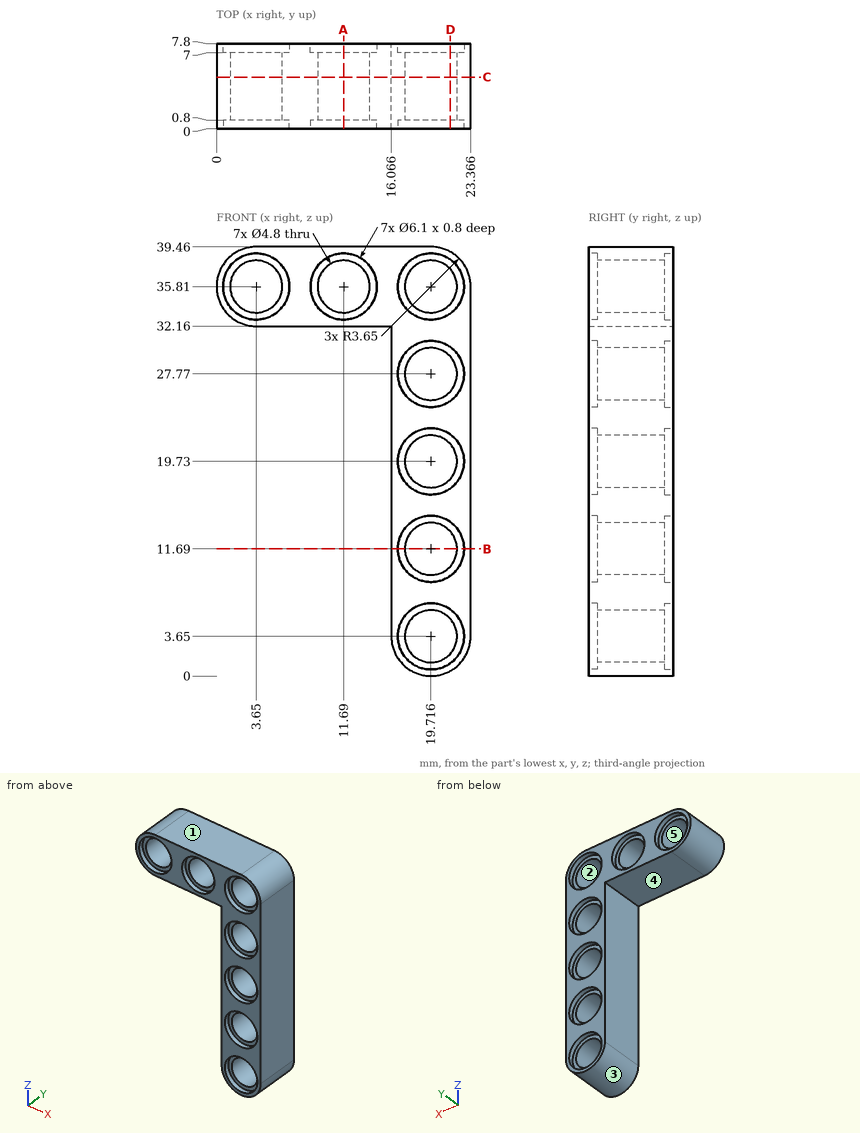
Answer from the drawing. Dimensions are ordinates in mm from the lowest x, y and z of the part. A direction names the side the tool comes from. Give positions to 0.01 mm unless a question says otherwise; leave off trailing zeros. Loops run counter-clockwise (first coordinate to the right, second up) from the corner with the lowest first, then second, coordinate; pieces in that order, holes last. Notation, with made-up numbers: (-16, 2.5) - (18, 2.5) arc R14 ccw to (18, 13.5) - close; hole circle Ø5 at (66.25, 85.5). An arc over 180 degrees is marked (long way). Answer as CSV lines item,"result". Start each with the question number.
Item 1: For the marked faces 4 and 5, determine the directions among +Z, -Z, +X, -X, +Y, -Y from which every point of the face is accessible in a straight line to the end or side of a thin tool.
Item 2: A cutting plane is placed at D-D on x = 21.5. Count the separate pieces of the cut face and the enclosed holes in it, then the cut area to 3 significant figures.
Item 3: A cutting plane is placed at B-B on z = 11.69. Determine the outline of the cut face in (x, y).
Item 4: The mould has two halves that part along X. Classify the marked faces 1, 2 and 3: +X half, -X half, draft (parallel to the pull), parting line (faces both ways), or undercut.
Item 5: A cutting plane is placed at C-C on y = 4.75. Determine the outline of the cut face in (x, z), then the cut area to 3 significant figures.
Item 6: A cutting plane is placed at A-A on x = 11.69. Determine the outline of the cut face in (y, z).
Item 7: Find the intervals of material crossed by line 1 (X direction, y = 7.5, z = 35.81); line 2 (Z direction, x = 11.69, y = 2); line 3 (X direction, y = 7.3, z = 11.69), in increasing order. Write a range as from..to.
Item 8: Each of these flat-tipped pins is pushed along its axis until it touches: pin 1 (1.8 mm diameter, centred on x = 18.5, z = 37, fed in from -Y); pin 2 (3.5 mm diameter, centred on x = 19.72, z = 19.73, fed in from +Y); pin 3 (5 mm diameter, centred on x = 3.65, z = 35.81, fed in from +Y); pin 4 (2 mm diameter, centred on x = 16.5, y = 1, fed in from -Z). Where does it stop, or does it pass through?
Found:
1,face 4,"-Z, -X, +Y, -Y"
1,face 5,"+Y, -Y"
2,separate pieces,"6"
2,enclosed holes,"0"
2,area,"161 mm^2"
3,outline,"(16.07, 0) - (16.67, 0) - (16.67, 0.8) - (17.32, 0.8) - (17.32, 7) - (16.67, 7) - (16.67, 7.8) - (16.07, 7.8) - close; (22.12, 0.8) - (22.77, 0.8) - (22.77, 0) - (23.37, 0) - (23.37, 7.8) - (22.77, 7.8) - (22.77, 7) - (22.12, 7) - close"
4,face 1,"draft"
4,face 2,"undercut"
4,face 3,"parting line"
5,outline,"(3.65, 32.16) - (16.07, 32.16) - (16.07, 3.65) arc R3.65 ccw to (23.37, 3.65) - (23.37, 35.81) arc R3.65 ccw to (19.72, 39.46) - (3.65, 39.46) arc R3.65 ccw to start; hole circle Ø4.8 at (3.65, 35.81); hole circle Ø4.8 at (11.69, 35.81); hole circle Ø4.8 at (19.72, 3.65); hole circle Ø4.8 at (19.72, 11.69); hole circle Ø4.8 at (19.72, 19.73); hole circle Ø4.8 at (19.72, 27.77); hole circle Ø4.8 at (19.72, 35.81)"
5,area,"264 mm^2"
6,outline,"(0, 32.16) - (7.8, 32.16) - (7.8, 32.76) - (7, 32.76) - (7, 33.41) - (0.8, 33.41) - (0.8, 32.76) - (0, 32.76) - close; (0, 38.86) - (0.8, 38.86) - (0.8, 38.21) - (7, 38.21) - (7, 38.86) - (7.8, 38.86) - (7.8, 39.46) - (0, 39.46) - close"
7,line 1,"x = 0..0.6, 6.7..8.64, 14.74..16.67, 22.77..23.37"
7,line 2,"z = 32.16..33.41, 38.21..39.46"
7,line 3,"x = 16.07..16.67, 22.77..23.37"
8,pin 1,"stops at y = 0.8"
8,pin 2,"passes through"
8,pin 3,"stops at y = 7"
8,pin 4,"stops at z = 0.75"
